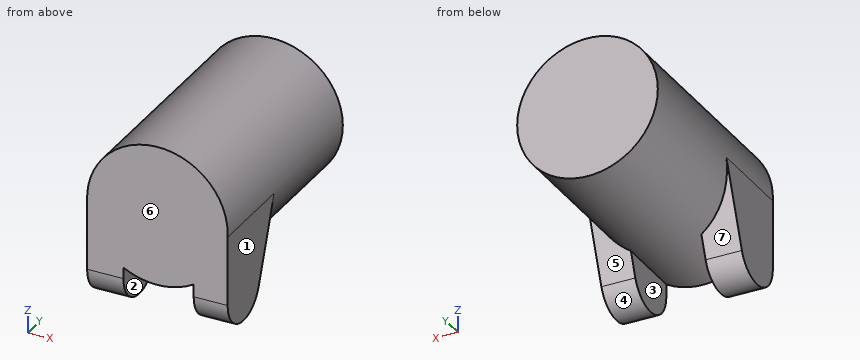
```python
from build123d import *

# Parameters (mm, degrees)
F1_DEPTH = 50.8
F2_W     = 50.8
F2_H     = 74.168
F3_DEPTH = 170.688
F4_R     = 50.8571740797
F5_DEPTH = 159.258


with BuildPart() as f1:
    # F0 (on Right) → F1 (new body, symmetric)
    with BuildSketch(Plane.YZ):
        with BuildLine():
            Line((0, 40.3383746743), (0, -11.3177125019))
            ThreePointArc((0, -11.3177125019), (18.2004266595, -33.0743933699), (42.8294130616, -19.0023742616))
            Line((42.8294130616, -19.0023742616), (64.8321659319, 40.3383746743))
            Line((64.8321659319, 40.3383746743), (0, 40.3383746743))
        make_face()
    extrude(amount=F1_DEPTH, both=True)

    # F2 (on Front) → F3 (cut)
    with BuildSketch(Plane.XZ):
        with Locations((0.8334377781, 3.3744326594)):
            Rectangle(F2_W, F2_H)
    extrude(amount=-F3_DEPTH, mode=Mode.SUBTRACT)

    # F4 (on Front) → F5 (join)
    with BuildSketch(Plane.XZ):
        with Locations((0, 41.3384996355)):
            Circle(F4_R)
    extrude(amount=-F5_DEPTH)


solid = f1.part
```
Source: CAD feature listing. Evaluate the final solid. Frame: model axes, mm. Face numbers are marked on the shaded views. A direction names the side the tool comes from. Round coordinates to 2 decimals unless told otherwise and drop trailing zeros. Loops run counter-clockwise (first coordinate to the right, second up) from the corner with the lowest first, then second, coordinate; pieces in that order, holes last.
(1) Pull-direction query (X, two-part tool) for the marked faces 1, 2, 3 and 4; classes: +X half, -X half, draft (parallel to the pull), parting line (faces both ways), or undercut.
From the geometry:
face 1: +X half
face 2: undercut
face 3: undercut
face 4: draft
(2) Section query D-D (x = 0). Output: boundary loops of the cut face in (y, z).
From the geometry:
outline: (0, -9.52) - (159.26, -9.52) - (159.26, 92.2) - (0, 92.2) - close
(3) Section query B-B (z = 9.5). Output: boundary loops of the cut face in (x, y), and give its area (3 significant figures).
From the geometry:
outline: (-50.8, 0) - (50.8, 0) - (50.8, 53.4) - (39.66, 53.4) - (39.66, 159.26) - (-39.66, 159.26) - (-39.66, 53.4) - (-50.8, 53.4) - close
area: 13,800 mm2
(4) Contact query for flat-ended pins moving along their axis: pin 1 Ø1 at (x, y) = (-32.5, 126.5) entering from +Z; pin 2 Ø19.5 at (y, z) = (41.5, 13) entering from -X; pin 3 Ø12 at (x, y) = (-7, 70.5) entering from +Z. Output: stop coordinate, or through.
From the geometry:
pin 1: stops at z = 80.87
pin 2: stops at x = -50.8
pin 3: stops at z = 92.19
(5) Section query C-C (y = 127). Output: boundary loops of the cut face in (x, z).
From the geometry:
outline: circle Ø101.71 at (0, 41.34)
(6) Access query for the marked faces 5, 6 and 7. Directions: +Z, -Z, +X, -X, +Y, -Y. A direction counts if a zero-diameter tool reaches every point of the face in a straight line with its end or side. Return the directions, or none.
From the geometry:
face 5: -Z, +X, +Y
face 6: +Z, -Z, +X, -X, -Y
face 7: -Z, -X, +Y
(7) Section query A-A (x = 37). Output: boundary loops of the cut face in (y, z).
From the geometry:
outline: (0, -11.32) arc R22.1 ccw to (42.83, -19) - (52.27, 6.45) - (159.26, 6.45) - (159.26, 76.23) - (0, 76.23) - close
(8) Material intervals for probe 1 along X at (y, z) = (37, 43.5); probe 2 along X at (y, z) = (22.5, 46); probe 3 along Y at (x, z) = (34, -2.5), sorted ascending.
From the geometry:
probe 1: x = -50.81 to 50.81
probe 2: x = -50.64 to 50.64
probe 3: y = 0 to 48.95
